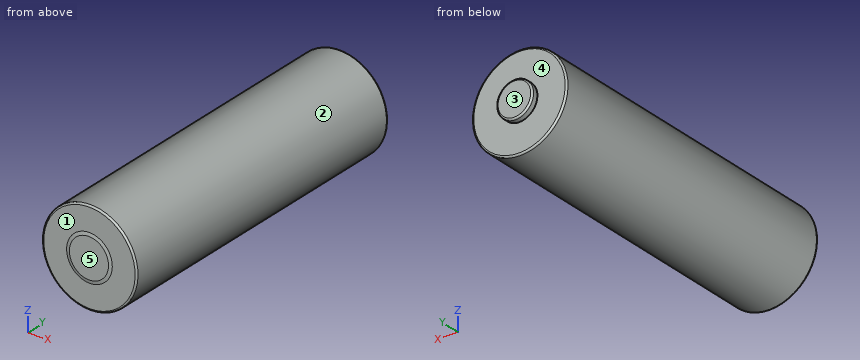
from build123d import *


with BuildPart() as part:
    # Sketch2 → Revolve1 (revolve)
    with BuildSketch(Plane(origin=(0, 0, 0), x_dir=(0, 0, -1), z_dir=(1, 0, 0))):
        with BuildLine():
            Line((0, 0), (0, 50.5))
            Line((0, 50.5), (2.5, 50.5))
            ThreePointArc((2.5, 50.5), (2.676776695, 50.426776695), (2.75, 50.25))
            Line((2.75, 50.25), (2.75, 49.5))
            Line((2.75, 49.5), (7, 49.5))
            ThreePointArc((7, 49.5), (7.176776695, 49.426776695), (7.25, 49.25))
            Line((7.25, 49.25), (7.25, 0.35))
            ThreePointArc((7.25, 0.35), (7.176776695, 0.173223305), (7, 0.1))
            Line((7, 0.1), (3.5, 0.1))
            Line((3.5, 0.1), (3, 0))
            Line((3, 0), (0, 0))
        make_face()
    revolve(axis=Axis((0, 0, 0), (0, -1, 0)))


solid = part.part
Can you work these out from the model? Positions are in its coordinate system, mm. Face numbers are marked on the shaded views. A direction names the side the tool comes from. Coordinates: 2 decimals unless noted, no trailing zeros. Loops run counter-clockwise (first coordinate to the right, second up) from the corner with the lowest first, then second, coordinate; pieces in that order, holes last. Notation, with made-up numbers: M 54,-26 L 94,-26 A22 ccw 94,-2 Z; hole C 50,-8.75 d2. An arc over 180 degrees is marked long. Return JSON: item names as keys, results as strings. Group by question number.
Item 1: On a 3-axis mill with a long thin cutter (end or side, diameter ignored), from which of +Z, -Z, +X, -X, +Y, -Y can I reach the whole of each face in a straight line? I mean the marked faces 4 and 5. Say none if no direction works.
Item 2: I'm going to push flat-ended pins straight in: pin 1 Ø1.5 at (x, y) = (-2.5, 9.5) entering from -Z; pin 2 Ø3 at (y, z) = (15.5, 2) entering from +X; pin 3 Ø1 at (x, y) = (-4, 23.5) entering from -Z. Where does each tip first touch, or does it pass through?
Item 3: Imagine slicing it at A-A (y = 7.5). Please give me the cut outline in (x, z), and give its area (3 significant figures).
Item 4: Thinking about a two-plate mould opening in Y: for the marked faces 1, 2 and 3, which applies, released by +Y, released by -Y, zero draft, split by the parting line, or undercut?
Item 5: If I drill on L1, parallel to Y at x = -2.5, z = -6.25; L2, parallel to Y at x = -0.5, z = 3; L3, parallel to Z at x = 3, y = 4, over which ranges is the centre line in solid material (lowest first)? Write a range as from..to.
Verdict:
{
 "1": {"face 4": "+Y", "face 5": "+Z, -Z, +X, -X, -Y"},
 "2": {"pin 1": "stops at z = -7.04", "pin 2": "stops at x = 7.23", "pin 3": "stops at z = -6.35"},
 "3": {"outline": "C 0,0 d14.5", "area": "165 mm^2"},
 "4": {"face 1": "released by -Y", "face 2": "zero draft", "face 3": "released by +Y"},
 "5": {"L1": "y = 0.1..49.5", "L2": "y = 0.01..49.5", "L3": "z = -6.6..6.6"}
}
